Verification items for the finished model (mm, model axes). A direction names the side the tool comes from. Give positions to 0.01 mm unless a question says otherwise; leave off trailing zeros. Write each loop counter-clockwise with the first axis right and the second up, starting at its lowest first coordinate (ties: lowest second). Pieces come first, ordered by that corner, then holes. Notation, with made-up numbers: (-7.5, -32) -> (-1.5, -32) arc R14 ccw to (-1.5, -13) -> close; hole circle Ø6 at (-20, 54.5). An arc over 180 degrees is marked (long way). Answer as CSV lines item,"result". Start each with the question number.
1) Sectioned sample at A-A on x = 5.5. Record the cut outline in (y, z), and give its area (4 significant figures).
2) Tool access check on faces 5 (the flat face through (-15, -21, 2)), 6 (the flat face through (0, -18, 16)), 7 (the flat face through (0, -15, 15)), 8 (the cylindrical face through (19.43, 15.6, 17.26)). Record the directions out of +Z, -Z, +X, -X, +Y, -Y that give a thin tool (end or side, any length) a straight path to the whole face; none if there is none.
3) Material ranges on L1, parallel to Z at x = 7.5, y = 19; L2, parallel to Y at x = -14.5, z = 3.5; L3, parallel to Y at x = 13, z = 15.5, recorded low to high.
4) Mould release check, pull along Y, two halves, no side actions. Record for faces 1 (the flat face through (0, 21, 3)), 2 (the flat face through (0, 0, 1.5)), 3 (the cylindrical face through (-19.4, -15.57, 15.26)), 4 (the flat face through (0, 21.5, 9)): released by +Y, released by -Y, zero draft, split by the parting line, or undercut.
5) Sectioned sample at D-D on z = 10. Record the cut outline in (x, y).
6) Sectioned sample at C-C on y = -17.5. Record the cut outline in (x, z), and give its area (3 significant figures).
7) Sectioned sample at B-B on z = 15. Record the cut outline in (x, y), and give its area (3 significant figures).
8) Gauge pin test, flat ends, axial feed: pin 1 Ø5 at (x, y) = (8, -18.5) entering from +Z; pin 2 Ø0.8 at (x, z) = (-3, 17) entering from -Y; pin 3 Ø12 at (x, y) = (-10, -4.5) entering from +Z. Record the tip position at first contact, or that the pin passes through.
```python
from build123d import *

# Parameters (mm, degrees)
F0_W      = 40
F0_H      = 43
F1_DEPTH  = 1.5
F2_W      = 40
F2_H      = 1.5
F3_DEPTH  = 14.5
F4_W      = 40
F4_H      = 1.5
F5_DEPTH  = 16.5
F6_W      = 40
F6_H      = 1.5
F7_DEPTH  = 5
F8_W      = 40
F8_H      = 1.5
F9_DEPTH  = 5
F10_W     = 30
F10_H     = 1.5
F11_DEPTH = 44
F12_R     = 2


with BuildPart() as f1:
    # F0 (on Top) → F1 (new body)
    with BuildSketch(Plane.XY):
        Rectangle(F0_W, F0_H)
    extrude(amount=F1_DEPTH)

    # F2 (on face) → F3 (join)
    with BuildSketch(Plane.XY.offset(1.5)):
        with Locations((0, -20.75)):
            Rectangle(F2_W, F2_H)
    extrude(amount=F3_DEPTH)

    # F4 (on face) → F5 (join)
    with BuildSketch(Plane.XY.offset(1.5)):
        with Locations((0, 20.75)):
            Rectangle(F4_W, F4_H)
    extrude(amount=F5_DEPTH)

    # F6 (on face) → F7 (join)
    with BuildSketch(Plane.XZ.offset(-20)):
        with Locations((0, 17.25)):
            Rectangle(F6_W, F6_H)
    extrude(amount=F7_DEPTH)

    # F8 (on face) → F9 (join)
    with BuildSketch(Plane(origin=(0, -20, 0), x_dir=(-1, 0, 0), z_dir=(0, 1, 0))):
        with Locations((0, 15.25)):
            Rectangle(F8_W, F8_H)
    extrude(amount=F9_DEPTH)

    # F10 (on face) → F11 (cut)
    with BuildSketch(Plane.XZ.offset(21.5)):
        with Locations((0, 2.25)):
            Rectangle(F10_W, F10_H)
    extrude(amount=-F11_DEPTH, mode=Mode.SUBTRACT)

    # F12
    f12_edges = [f1.edges().sort_by_distance(p)[0] for p in [
        (20, 15, 17.25),
        (20, -15, 15.25),
        (-20, 15, 17.25),
        (-20, -15, 15.25),
    ]]
    fillet(f12_edges, radius=F12_R)


solid = f1.part
```
Ans:
1,outline,"(-21.5, 0) -> (21.5, 0) -> (21.5, 1.5) -> (-21.5, 1.5) -> close; (-21.5, 3) -> (-20, 3) -> (-20, 14.5) -> (-15, 14.5) -> (-15, 16) -> (-21.5, 16) -> close; (15, 16.5) -> (20, 16.5) -> (20, 3) -> (21.5, 3) -> (21.5, 18) -> (15, 18) -> close"
1,area,"121.5 mm²"
2,face 5,"+Y, -Y"
2,face 6,"+Z, +X, -X, -Y"
2,face 7,"+Z, +X, -X"
2,face 8,"+Z, +X, -Y"
3,L1,"z = 0 to 1.5, 16.5 to 18"
3,L2,"y = -21.5 to -20, 20 to 21.5"
3,L3,"y = -21.5 to -15, 20 to 21.5"
4,face 1,"zero draft"
4,face 2,"undercut"
4,face 3,"undercut"
4,face 4,"released by +Y"
5,outline,"(-20, -21.5) -> (20, -21.5) -> (20, -20) -> (-20, -20) -> close; (-20, 20) -> (20, 20) -> (20, 21.5) -> (-20, 21.5) -> close"
6,outline,"(-20, 0) -> (20, 0) -> (20, 1.5) -> (-20, 1.5) -> close; (-20, 14.5) -> (20, 14.5) -> (20, 16) -> (-20, 16) -> close"
6,area,"120 mm²"
7,outline,"(-20, -21.5) -> (20, -21.5) -> (20, -17) arc R2 ccw to (18, -15) -> (-18, -15) arc R2 ccw to (-20, -17) -> close; (-20, 20) -> (20, 20) -> (20, 21.5) -> (-20, 21.5) -> close"
7,area,"318 mm²"
8,pin 1,"stops at z = 16"
8,pin 2,"stops at y = 15"
8,pin 3,"stops at z = 1.5"
